The listing builds one solid part. Answer for the finished solid, in the listing's coordinates (mm). A direction names the side the tool comes from. Coordinates: 2 decimals unless noted, no trailing zeros. Write each loop counter-clockwise with the first axis right and the second up, starting at its lowest first coordinate (ties: lowest second). Pieces come first, ordered by that corner, then holes. Notation, with made-up numbers: M 75.5,-10 L 134.5,-10 A29 ccw 134.5,15 Z; hole C -31,19.5 d1. An arc over 180 degrees is marked long. Answer as a JSON object with one key per item and string values. Group by question number.
from build123d import *

# Parameters (mm, degrees)
BOSS_EXTRUDE1_DEPTH            = 50
SKETCH4_W                      = 15
SKETCH4_H                      = 11.826160891
CUT_EXTRUDE3_DEPTH             = 17
SKETCH5_R                      = 2.5
CUT_EXTRUDE4_DEPTH             = 17
CUT_EXTRUDE4_DEPTH_BACK        = 24
SKETCH9_W                      = 25
SKETCH9_H                      = 11.826160891
CUT_EXTRUDE8_DEPTH             = 17
CUT_EXTRUDE8_DEPTH_BACK        = 24
CUT_EXTRUDE9_REACH             = 44
CUT_EXTRUDE9_DIRECTION_2_REACH = 16.792
CUT_EXTRUDE10_DEPTH            = 13
CUT_EXTRUDE10_DEPTH_BACK       = 13.5000001
CUT_EXTRUDE11_DEPTH            = 20.5
CUT_EXTRUDE11_DEPTH_BACK       = 20.5
CUT_EXTRUDE15_REACH            = 58.792
SKETCH14_R                     = 3.375
BOSS_EXTRUDE2_DEPTH            = 2.5
CUT_EXTRUDE17_DEPTH            = 25
SKETCH16_W                     = 20
SKETCH16_H                     = 25
CUT_EXTRUDE18_DEPTH            = 0.5


with BuildPart() as part:
    # Sketch1 → Boss-Extrude1 (new body)
    with BuildSketch(Plane.XY):
        with BuildLine():
            Line((3.5, 29.291637032), (1, 29.291637032))
            Line((1, 29.291637032), (1, 14.465476141))
            ThreePointArc((1, 14.465476141), (0, -14.5), (-1, 14.465476141))
            Line((-1, 14.465476141), (-1, 29.291637032))
            Line((-1, 29.291637032), (-3.5, 29.291637032))
            Line((-3.5, 29.291637032), (-16.058186159, 11.06275993))
            ThreePointArc((-16.058186159, 11.06275993), (-19.250030671, -3.112285199), (-11.754006256, -15.559348859))
            ThreePointArc((-11.754006256, -15.559348859), (-6.198495674, -18.488608692), (0, -19.5))
            ThreePointArc((0, -19.5), (6.13886546, -18.508493479), (11.653451419, -15.634803166))
            ThreePointArc((11.653451419, -15.634803166), (12.039474024, -15.299956246), (12.455712019, -15.003507527))
            ThreePointArc((12.455712019, -15.003507527), (17.651294349, -8.287448812), (19.5, 0))
            ThreePointArc((19.5, 0), (18.269595128, 6.817029694), (14.733651913, 12.773781793))
            Line((14.733651913, 12.773781793), (3.5, 29.291637032))
        make_face()
        with BuildLine():
            ThreePointArc((10, -19.5), (10.430719001, -17.397998087), (11.653451419, -15.634803166))
            ThreePointArc((11.653451419, -15.634803166), (6.13886546, -18.508493479), (0, -19.5))
            ThreePointArc((0, -19.5), (-6.198495674, -18.488608692), (-11.754006256, -15.559348859))
            ThreePointArc((-11.754006256, -15.559348859), (-10.458303194, -17.343308705), (-10, -19.5))
            Line((-10, -19.5), (-10, -27.5))
            Line((-10, -27.5), (10, -27.5))
            Line((10, -27.5), (10, -19.5))
        make_face()
    extrude(amount=-BOSS_EXTRUDE1_DEPTH)

    # Sketch4 → Cut-Extrude3 (cut, through all)
    with BuildSketch(Plane(origin=(3.5, 0, 0), x_dir=(0, 0, -1), z_dir=(1, 0, 0))):
        with Locations((12.5, 23.378556587)):
            Rectangle(SKETCH4_W, SKETCH4_H)
    cut_extrude3 = extrude(amount=CUT_EXTRUDE3_DEPTH, mode=Mode.SUBTRACT)

    # Mirror1: Cut-Extrude3 across plane
    add(cut_extrude3.mirror(Plane(origin=(0, 0, 0), x_dir=(0, 0, 1), z_dir=(1, 0, 0))), mode=Mode.SUBTRACT)

    # Sketch5 → Cut-Extrude4 (cut, two sides)
    with BuildSketch(Plane(origin=(3.5, 0, 0), x_dir=(0, 0, -1), z_dir=(1, 0, 0))) as cut_extrude4_sk:
        with Locations((12.5, 23.378556587)):
            Circle(SKETCH5_R)
    extrude(amount=CUT_EXTRUDE4_DEPTH, mode=Mode.SUBTRACT)
    extrude(cut_extrude4_sk.sketch, amount=-CUT_EXTRUDE4_DEPTH_BACK, mode=Mode.SUBTRACT)

    # Sketch9 → Cut-Extrude8 (cut, two sides)
    with BuildSketch(Plane(origin=(3.5, 0, 0), x_dir=(0, 0, -1), z_dir=(1, 0, 0))) as cut_extrude8_sk:
        with Locations((37.5, 23.378556587)):
            Rectangle(SKETCH9_W, SKETCH9_H)
    extrude(amount=CUT_EXTRUDE8_DEPTH, mode=Mode.SUBTRACT)
    extrude(cut_extrude8_sk.sketch, amount=-CUT_EXTRUDE8_DEPTH_BACK, mode=Mode.SUBTRACT)

    # Sketch8 → Cut-Extrude9 (cut, up to next)
    with BuildSketch(Plane(origin=(0, 14.5, 0), x_dir=(1, 0, 0), z_dir=(0, 1, 0)), mode=Mode.PRIVATE) as cut_extrude9_sk1:
        with BuildLine():
            Line((-10.5, 37.5), (-10.5, 50))
            Line((-10.5, 50), (-1, 50))
            Line((-1, 50), (-1, 27.04772752))
            ThreePointArc((-1, 27.04772752), (-7.770135134, 30.437776554), (-10.5, 37.5))
        make_face()
    cut_extrude9_tool1 = extrude(cut_extrude9_sk1.sketch, amount=-CUT_EXTRUDE9_REACH, mode=Mode.PRIVATE) & part.part
    add(cut_extrude9_tool1.solids().sort_by_distance((-5.457616, 14.5, -39.610639))[0], mode=Mode.SUBTRACT)
    # Sketch8 → Cut-Extrude9 (cut, up to next)
    with BuildSketch(Plane(origin=(0, 14.5, 0), x_dir=(1, 0, 0), z_dir=(0, 1, 0)), mode=Mode.PRIVATE) as cut_extrude9_sk2:
        with BuildLine():
            Line((10.5, 50), (10.5, 37.5))
            ThreePointArc((10.5, 37.5), (7.770135134, 30.437776554), (1, 27.04772752))
            Line((1, 27.04772752), (1, 50))
            Line((1, 50), (10.5, 50))
        make_face()
    cut_extrude9_tool2 = extrude(cut_extrude9_sk2.sketch, amount=-CUT_EXTRUDE9_REACH, mode=Mode.PRIVATE) & part.part
    add(cut_extrude9_tool2.solids().sort_by_distance((5.457616, 14.5, -39.610639))[0], mode=Mode.SUBTRACT)

    # Sketch8 → Cut-Extrude9 direction 2 (cut, up to next)
    with BuildSketch(Plane(origin=(0, 14.5, 0), x_dir=(1, 0, 0), z_dir=(0, 1, 0)), mode=Mode.PRIVATE) as cut_extrude9_direction_2_sk1:
        with BuildLine():
            Line((-10.5, 37.5), (-10.5, 50))
            Line((-10.5, 50), (-1, 50))
            Line((-1, 50), (-1, 27.04772752))
            ThreePointArc((-1, 27.04772752), (-7.770135134, 30.437776554), (-10.5, 37.5))
        make_face()
    cut_extrude9_direction_2_tool1 = extrude(cut_extrude9_direction_2_sk1.sketch, amount=CUT_EXTRUDE9_DIRECTION_2_REACH, mode=Mode.PRIVATE) & part.part
    add(cut_extrude9_direction_2_tool1.solids().sort_by_distance((-5.457616, 14.5, -39.610639))[0], mode=Mode.SUBTRACT)
    # Sketch8 → Cut-Extrude9 direction 2 (cut, up to next)
    with BuildSketch(Plane(origin=(0, 14.5, 0), x_dir=(1, 0, 0), z_dir=(0, 1, 0)), mode=Mode.PRIVATE) as cut_extrude9_direction_2_sk2:
        with BuildLine():
            Line((10.5, 50), (10.5, 37.5))
            ThreePointArc((10.5, 37.5), (7.770135134, 30.437776554), (1, 27.04772752))
            Line((1, 27.04772752), (1, 50))
            Line((1, 50), (10.5, 50))
        make_face()
    cut_extrude9_direction_2_tool2 = extrude(cut_extrude9_direction_2_sk2.sketch, amount=CUT_EXTRUDE9_DIRECTION_2_REACH, mode=Mode.PRIVATE) & part.part
    add(cut_extrude9_direction_2_tool2.solids().sort_by_distance((5.457616, 14.5, -39.610639))[0], mode=Mode.SUBTRACT)

    # Sketch10 → Cut-Extrude10 (cut, two sides)
    with BuildSketch(Plane.XY.offset(-37.5)) as cut_extrude10_sk:
        with BuildLine():
            Line((-7, -12.698425099), (7, -12.698425099))
            Line((7, -12.698425099), (7, -14.941552797))
            ThreePointArc((7, -14.941552797), (0, -16.5), (-7, -14.941552797))
            Line((-7, -14.941552797), (-7, -12.698425099))
        make_face()
    extrude(amount=CUT_EXTRUDE10_DEPTH, mode=Mode.SUBTRACT)
    extrude(cut_extrude10_sk.sketch, amount=-CUT_EXTRUDE10_DEPTH_BACK, mode=Mode.SUBTRACT)

    # Sketch11 → Cut-Extrude11 (cut, two sides)
    with BuildSketch(Plane(origin=(0, 0, 0), x_dir=(0, 0, -1), z_dir=(1, 0, 0))) as cut_extrude11_sk:
        Polygon((5, -7.5), (0, -10), (0, 10), (5, 7.5), align=None)
    extrude(amount=CUT_EXTRUDE11_DEPTH, mode=Mode.SUBTRACT)
    extrude(cut_extrude11_sk.sketch, amount=-CUT_EXTRUDE11_DEPTH_BACK, mode=Mode.SUBTRACT)

    # Sketch13 → Cut-Extrude15 (cut, up to next)
    with BuildSketch(Plane.XZ.offset(27.5), mode=Mode.PRIVATE) as cut_extrude15_sk1:
        Polygon((0, -31.084195134), (-5.55625, -34.292097567), (-5.55625, -40.707902433), (0, -43.915804866), (5.55625, -40.707902433), (5.55625, -34.292097567), align=None)
    cut_extrude15_tool1 = extrude(cut_extrude15_sk1.sketch, amount=-CUT_EXTRUDE15_REACH, mode=Mode.PRIVATE) & part.part
    add(cut_extrude15_tool1.solids().sort_by_distance((0, -27.5, -37.5))[0], mode=Mode.SUBTRACT)

    # Sketch14 → Boss-Extrude2 (add)
    with BuildSketch(Plane.XZ.offset(27.5)):
        Polygon((5.55625, -40.707902433), (5.55625, -34.292097567), (0, -31.084195134), (-5.55625, -34.292097567), (-5.55625, -40.707902433), (0, -43.915804866), align=None)
        with Locations((0, -37.5)):
            Circle(SKETCH14_R, mode=Mode.SUBTRACT)
    extrude(amount=-BOSS_EXTRUDE2_DEPTH)

    # Sketch15 → Cut-Extrude17 (cut)
    with BuildSketch(Plane.XY):
        with BuildLine():
            Line((-19.5, 0), (-19.5, -27.5))
            Line((-19.5, -27.5), (19.5, -27.5))
            Line((19.5, -27.5), (19.5, 0))
            ThreePointArc((19.5, 0), (0, -19.5), (-19.5, 0))
        make_face()
    extrude(amount=-CUT_EXTRUDE17_DEPTH, mode=Mode.SUBTRACT)

    # Sketch16 → Cut-Extrude18 (cut)
    with BuildSketch(Plane.XZ.offset(27.5)):
        with Locations((0, -37.5)):
            Rectangle(SKETCH16_W, SKETCH16_H)
    extrude(amount=-CUT_EXTRUDE18_DEPTH, mode=Mode.SUBTRACT)


solid = part.part
Item 1: A cutting plane is placed at B-B, the plane z = -22. Write down the section's boundary in (x, y), and give its area (3 significant figures).
Item 2: A cutting plane is placed at C-C, the plane y = 5. Write down the section's boundary in (x, z), and give its area (3 significant figures).
Item 3: Flat-ended cylindrical pins translate along their axes: pin 1 Ø5.5 at (x, z) = (-7, -33.5) entering from +Y; pin 2 Ø0.7 at (y, z) = (-14, -32) entering from +X; pin 3 Ø1.5 at (y, z) = (-3.5, -40) entering from -X. Find the tip coordinate at first contact, or state that the pin passes through.
Item 4: A cutting plane is placed at A-A, the plane z = -12.5. Write down the section's boundary in (x, y).
Item 5: For a pull along X with two mould halves and no side action, classify faces 5 (the face through (-9, 17.465, -31)), 6 (the face through (3.5, 26, -12)), 7 (the face through (-10.5, 14, -44)), 8 (the face through (7, -14, -37)) as +X half, -X half, draft (parallel to the pull), parting line (faces both ways), or undercut.
Item 6: Consider L1, parallel to Y at x = -2.25, z = -12.5; L2, parallel to Z at x = 0, y = -25.7 (3 decimals); L3, parallel to X at y = 0, z = -22. Determine where each line is inside the solid, lowest interval first. Write a range as from..to.
Item 7: A tool of negligible diameter and unlimited length cuts with its end or side. For faces 1 (the face through (7, 17.465, -12)), 2 (the face through (-8.76, 14.61, -31.71)), 3 (the face through (1, 20, -13)), 4 (the face through (-7, 22, -5)), from which of +Z, -Z, +X, -X, +Y, -Y can it reach the whole face along a straight path? Write none if from no direction.
Item 8: A cutting plane is placed at D-D, the plane x = 16. Write down the section's boundary in (y, z), and give its area (3 significant figures).
Answer:
{
 "1": {"outline": "M -16.06,11.06 A19.5 ccw 11.65,-15.63 A5.34 cw 12.46,-15 A19.5 ccw 14.73,12.77 L 3.5,29.29 L 1,29.29 L 1,14.47 A14.5 cw long -1,14.47 L -1,29.29 L -3.5,29.29 Z", "area": "669 mm2"},
 "2": {"outline": "M -18.85,-50 L -13.61,-50 L -13.61,-5 L -18.85,-5 Z; M 13.61,-50 L 18.85,-50 L 18.85,-5 L 13.61,-5 Z", "area": "471 mm2"},
 "3": {"pin 1": "y = 17.47", "pin 2": "x = 13.93", "pin 3": "x = -19.31"},
 "4": {"outline": "M -16.06,11.06 A19.5 ccw 11.65,-15.63 A5.34 cw 12.46,-15 A19.5 ccw 14.73,12.77 L 11.54,17.47 L 3.5,17.47 L 3.5,20.88 L 1,20.88 L 1,14.47 A14.5 cw long -1,14.47 L -1,20.88 L -3.5,20.88 L -3.5,17.47 L -11.65,17.47 Z; M -3.5,25.88 L -1,25.88 L -1,29.29 L -3.5,29.29 Z; M 1,25.88 L 3.5,25.88 L 3.5,29.29 L 1,29.29 Z"},
 "5": {"face 5": "draft", "face 6": "+X half", "face 7": "undercut", "face 8": "undercut"},
 "6": {"L1": "-19.37..-14.32, 14.32..20.88, 25.88..29.29", "L2": "-50..-40.875, -34.125..-25", "L3": "-19.5..-14.5, 14.5..19.5"},
 "7": {"face 1": "+X, +Y", "face 2": "-Z, +Y", "face 3": "+Z, -Z, +Y", "face 4": "-X, +Y"},
 "8": {"outline": "M -11.15,-50 L 11.15,-50 L 11.15,0 L 10,0 L 7.5,-5 L -7.5,-5 L -10,0 L -11.15,0 Z", "area": "1,030 mm2"}
}
